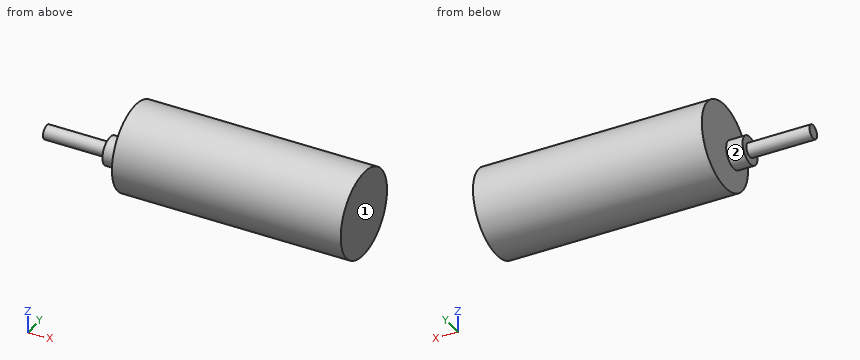
Autodesk Inventor part; units mm, degrees
ref_plane "YZ Plane" through (0, 0, 0) normal (1, 0, 0) x (0, 1, 0)
ref_plane "XZ Plane" through (0, 0, 0) normal (0, 1, 0) x (-1, 0, 0)
ref_plane "XY Plane" through (0, 0, 0) normal (0, 0, 1) x (1, 0, 0)
sketch "Sketch1" plane through (0, 0, 0) normal (0, 0, 1) x (1, 0, 0)
  line L0 (-46.4617, 18.5) -> (51.3383, 18.5)
  line L1 (51.3383, 18.5) -> (51.3383, 0)
  line L2 (-46.4617, 18.5) -> (-46.4617, 0)
  line L3 (-46.4617, 0) -> (51.3383, 0)
  point P0 (0, 0)
  dimension "d30" = 97.8
revolve "Revolution1" add sketch "Sketch1" angle 360 about axis through (-46.4617, 0, 0) along (1, 0, 0)
sketch "Sketch4" plane through (-46.4617, 0, 0) normal (-1, 0, 0) x (0, 0, 1)
  circle A0 centre (0, -7) radius 6
  point P0 (0, 0)
  dimension "d31" = 7
  dimension "d32" = 12
extrude "Extrusion3" add sketch "Sketch4" along normal blind 7
sketch "Sketch5" plane through (-53.4617, -7, 0) normal (-1, 0, 0) x (0, 0, 1)
  circle A0 centre (0, 0) radius 3
  point P0 (0, 7)
  dimension "d35" = 6
extrude "Extrusion4" add sketch "Sketch5" along normal blind 27
properties part number "Moteur"
Verification items for the finished model (mm, model axes). Face numbers are marked on the shaded views. A direction names the side the tool comes from. Coordinates: 2 decimals unless noted, no trailing zeros. Loops run counter-clockwise (first coordinate to the right, second up) from the corner with the lowest first, then second, coordinate; pieces in that order, holes last. Notation, with made-up numbers: (-31.75, 53.5) - (-6.75, 53.5) arc R16 cw to (-6.75, 80.5) - close; hole circle Ø4 at (45.25, 67). An arc over 180 degrees is marked (long way). Put each result on its own line as item: value.
Item 1: Section check B-B (x = 32.5). Enter the section's corners in (y, z), then the cut area to 3 significant figures.
Conclusion:
outline: circle Ø37 at (0, 0)
area: 1,080 mm2
Item 2: Section check D-D (z = 8.5). Enter the section's corners in (x, y).
Conclusion:
outline: (-46.46, -16.43) - (51.34, -16.43) - (51.34, 16.43) - (-46.46, 16.43) - close
Item 3: Section check A-A (z = 0). Enter the section's corners in (x, y), then the cut area to 3 significant figures.
Conclusion:
outline: (-80.46, -10) - (-53.46, -10) - (-53.46, -13) - (-46.46, -13) - (-46.46, -18.5) - (51.34, -18.5) - (51.34, 18.5) - (-46.46, 18.5) - (-46.46, -1) - (-53.46, -1) - (-53.46, -4) - (-80.46, -4) - close
area: 3,860 mm2
Item 4: Scan lines: line 1 along X through (y, z) = (-2, 15.5); line 2 along Y through (x, z) = (16, 0.5); line 3 along Z through (x, y) = (-12.5, -4.5). Record each from-to range of solid material in increasing order.
Conclusion:
line 1: x = -46.46 to 51.34
line 2: y = -18.49 to 18.49
line 3: z = -17.94 to 17.94
Item 5: Set-up check for the marked faces 1 and 2: record each of +Z, -Z, +X, -X, +Y, -Y from which the full face is reachable in a straight line by a thin tool's end or side.
Conclusion:
face 1: +Z, -Z, +X, +Y, -Y
face 2: -X
Item 6: Gauge pin test, flat ends, axial feed: pin 1 Ø6 at (x, y) = (28.5, -7) entering from -Z; pin 2 Ø12 at (x, z) = (3.5, 1.5) entering from -Y; pin 3 Ø3 at (x, y) = (-27.5, 3.5) entering from -Z; pin 4 Ø2 at (x, y) = (-15.5, -4.5) entering from +Z. Record the tip position at first contact, or that the pin passes through.
Conclusion:
pin 1: stops at z = -18.06
pin 2: stops at y = -18.5
pin 3: stops at z = -18.39
pin 4: stops at z = 18.17
Item 7: Section check C-C (y = -7). Enter the section's corners in (x, z).
Conclusion:
outline: (-80.46, -3) - (-53.46, -3) - (-53.46, -6) - (-46.46, -6) - (-46.46, -17.12) - (51.34, -17.12) - (51.34, 17.12) - (-46.46, 17.12) - (-46.46, 6) - (-53.46, 6) - (-53.46, 3) - (-80.46, 3) - close
